Part model, mm, in its own coordinate system. A direction names the side the tool comes from. Coordinates: 2 decimals unless noted, no trailing zeros. Loops run counter-clockwise (first coordinate to the right, second up) from the corner with the lowest first, then second, coordinate; pieces in that order, holes last. Notation, with made-up numbers: M 71.25,34 L 111.25,34 A16 ccw 111.25,60 Z; hole C 39.25,10 d6. An arc over 180 degrees is marked long. Answer as a JSON object with one key per item and string values. Group by question number.
1. Saw through at B-B on y = -59. Write the cut outline in (x, z).
2. Drop flat-ended pins along their axis: pin 1 Ø5 at (y, z) = (-78.5, -24) entering from -X; pin 2 Ø4 at (x, y) = (66.5, 13) entering from -Z; pin 3 Ø1.5 at (x, y) = (12.5, 64) entering from +Z. Give the stop position or say it passes through.
3. Saw through at C-C on z = -50.8. Write the cut outline in (x, y).
4. Saw through at D-D on z = 22. Write the cut outline in (x, y).
5. Drill centre lines: L1, parallel to Y at x = 2.5, z = 25; L2, parallel to Y at x = 16, z = 23; L3, parallel to Z at x = 83, y = 39. Where is each one in solid material? Low to high.
6. Saw through at A-A on x = 26. Write the cut outline in (y, z) (1 decimal), then the cut area to 3 significant figures.
7. 3-axis set-ups, long thin cutter, end or side, ignore diameter. For faces 1 (the face through (-76.2, 0, 0)), 2 (the face through (189.97, -3.1, 0.69)): which of +Z, -Z, +X, -X, +Y, -Y reach the whole face in a straight line?
8. Mould opens along Z. For faces 3 (the face through (228.6, 0, 0)), 4 (the face through (-38.63, -3.1, 0.69)), 5 (the face through (75.13, -10.01, -19)) say: released by +Z, released by -Z, zero draft, split by the parting line, or undercut.
from build123d import *

# Parameters (mm, degrees)
SKETCH1_R                = 101.6
BOSS_EXTRUDE1_DEPTH      = 152.4
SKETCH3_R                = 33.3375
CUT_EXTRUDE1_DEPTH       = 210.453765781
CIRPATTERN1_COUNT        = 4
BOSS_EXTRUDE7_DEPTH      = 228.6
BOSS_EXTRUDE7_DEPTH_BACK = 76.2
SKETCH2_R                = 3.175


with BuildPart() as part:
    # Sketch1 → Boss-Extrude1 (new body)
    with BuildSketch(Plane(origin=(0, 0, 0), x_dir=(0, 0, -1), z_dir=(1, 0, 0))):
        with Locations(Location((0, 0, 0), (0, 0, 180))):
            Circle(SKETCH1_R)
    extrude(amount=BOSS_EXTRUDE1_DEPTH)

    # Sketch3 → Cut-Extrude1 (cut, through all)
    with BuildSketch(Plane(origin=(0, 0, 0), x_dir=(0, 0, -1), z_dir=(1, 0, 0))):
        with Locations(Location((50.8, 0, 0), (0, 0, 180))):
            Circle(SKETCH3_R)
    cut_extrude1 = extrude(amount=CUT_EXTRUDE1_DEPTH, mode=Mode.SUBTRACT)

    # CirPattern1: Cut-Extrude1 ×4 about axis
    cirpattern1_axis = Axis((0, 0, 0), (1, 0, 0))
    for i in range(1, CIRPATTERN1_COUNT):
        add(cut_extrude1.rotate(cirpattern1_axis, i * 360 / CIRPATTERN1_COUNT), mode=Mode.SUBTRACT)

    # Sketch2 → Boss-Extrude7 (add, two sides: drawn at the far end of the back side and taken through both)
    with BuildSketch(Plane(origin=(0, 0, 0), x_dir=(0, 0, -1), z_dir=(1, 0, 0)).offset(-BOSS_EXTRUDE7_DEPTH_BACK)):
        Circle(SKETCH2_R)
    extrude(amount=BOSS_EXTRUDE7_DEPTH + BOSS_EXTRUDE7_DEPTH_BACK)


solid = part.part
Outcome:
{
 "1": {"outline": "M 0,-82.71 L 152.4,-82.71 L 152.4,-32.31 L 0,-32.31 Z; M 0,32.31 L 152.4,32.31 L 152.4,82.71 L 0,82.71 Z"},
 "2": {"pin 1": "stops at x = 0", "pin 2": "stops at z = -101", "pin 3": "stops at z = 79.51"},
 "3": {"outline": "M 0,-87.99 L 152.4,-87.99 L 152.4,-33.34 L 0,-33.34 Z; M 0,33.34 L 152.4,33.34 L 152.4,87.99 L 0,87.99 Z"},
 "4": {"outline": "M 0,-99.19 L 152.4,-99.19 L 152.4,-75.85 L 0,-75.85 Z; M 0,-25.75 L 152.4,-25.75 L 152.4,-16.79 L 0,-16.79 Z; M 0,16.79 L 152.4,16.79 L 152.4,25.75 L 0,25.75 Z; M 0,75.85 L 152.4,75.85 L 152.4,99.19 L 0,99.19 Z"},
 "5": {"L1": "y = -98.48 to -72.85, -28.75 to -21.11, 21.11 to 28.75, 72.85 to 98.48", "L2": "y = -98.96 to -74.93, -26.67 to -18.4, 18.4 to 26.67, 74.93 to 98.96", "L3": "z = -93.82 to -31.18, 31.18 to 93.82"},
 "6": {"outline": "C 0,0 d203.2; hole C -50.8,0 d66.7; hole C 0,-50.8 d66.7; hole C 0,50.8 d66.7; hole C 50.8,0 d66.7", "area": "18,500 mm²"},
 "7": {"face 1": "+Z, -Z, -X, +Y, -Y", "face 2": "+X"},
 "8": {"face 3": "zero draft", "face 4": "split by the parting line", "face 5": "undercut"}
}
